Autodesk Fusion 360 part; units mm, degrees
sketch "Sketch1" plane through (0, 0, 0) normal (0, 0, 1) x (1, 0, 0)
  circle A0 centre (0, 0) radius 10
  dimension "d1" = 20
extrude "Extrude1" add sketch "Sketch1" along normal blind 3
sketch "Sketch2" plane through (0, 0, 3) normal (0, 0, 1) x (-1, 0, 0)
  circle A0 centre (0, 0) radius 10
  circle A1 centre (0, 0) radius 1.5
  dimension "d4" = 3
extrude "Extrude2" cut sketch "Sketch2" against normal blind 12 contours A1
sketch "Sketch3" plane through (0, 0, 3) normal (0, 0, 1) x (-1, 0, 0)
  circle A0 centre (0, 0) radius 1.5
  circle A1 centre (0, 0) radius 10
  circle A2 centre (-4.6093, 0.0139) radius 0.8
  dimension "d7" = 1.6
sketch "Sketch4" plane through (0, 0, 3) normal (0, 0, 1) x (-1, 0, 0)
  circle A0 centre (4.6091, 0) radius 0.8
  dimension "d8" = 1.6
extrude "Extrude3" cut sketch "Sketch3" sketch "Sketch4" against normal blind 3 contours A2 of sketch 2
CAD build for the part. Positions are in the model's coordinates, mm. Give positions to 0.01 mm unless a question says otherwise; leave off trailing zeros. Order: outer loops, then holes, each group sorted by start corner. A loop starts at its lowest first (then second) coordinate and runs counter-clockwise, first axis right, second up. Notation, with made-up numbers: (23.5, -11.75) - (46.5, -11.75) arc R18 cw to (46.5, -7.75) - close; hole circle Ø9 at (-17.75, -30). An arc over 180 degrees is marked (long way). Answer in a Markdown table with one row per item.
1. Flat gauge pin, fed straight in: pin 1 (1.3 mm diameter, centred on x = 4.61, y = -0.01, fed in from -Z). Where does the tip first touch, or does it go through?
Data:
| item | result |
|---|---|
| pin 1 | passes through |
2. Saw through at B-B, the plane y = 2.5. Give the cut face in (x, z), plus the area to 3 significant figures.
Data:
| item | result |
|---|---|
| outline | (-9.68, 0) - (9.68, 0) - (9.68, 3) - (-9.68, 3) - close |
| area | 58.1 mm² |
3. Probe probe 1 along Y at (x, z) = (0, 2.05); probe 2 along X at (y, z) = (-0.5, 1.8); probe 3 along Y at (x, z) = (1, 1.65). List the from-to ranges inside material, lowest first. Write a range as [from, to].
Data:
| item | result |
|---|---|
| probe 1 | y = [-10, -1.5], [1.5, 10] |
| probe 2 | x = [-9.99, -5.23], [-3.98, -1.41], [1.41, 3.97], [5.24, 9.99] |
| probe 3 | y = [-9.95, -1.12], [1.12, 9.95] |
4. Saw through at C-C, the plane z = 1.6. Give the cut face in (x, y), plus the area to 3 significant figures.
Data:
| item | result |
|---|---|
| outline | circle Ø20 at (0, 0); hole circle Ø1.6 at (-4.61, 0); hole circle Ø3 at (0, 0); hole circle Ø1.6 at (4.61, -0.01) |
| area | 303 mm² |
5. Saw through at D-D, the plane x = -6.25. Give the cut face in (y, z).
Data:
| item | result |
|---|---|
| outline | (-7.81, 0) - (7.81, 0) - (7.81, 3) - (-7.81, 3) - close |
6. Pull direction X, two halves, no side cores. Call faces 1 (the cylindrical face through (-2.17, 9.76, 1.48)), 2 (the cylindrical face through (1.5, -0.07, 1.52)), 3 (the flat face through (2, 0, 0)): pulls with the +X half, pulls with the -X half, needs draft (parallel to the pull), parting line crosses it, or undercut.
Data:
| item | result |
|---|---|
| face 1 | parting line crosses it |
| face 2 | undercut |
| face 3 | needs draft |
7. Saw through at A-A, the plane x = 0. Give the cut face in (y, z).
Data:
| item | result |
|---|---|
| outline | (-10, 0) - (-1.5, 0) - (-1.5, 3) - (-10, 3) - close; (1.5, 0) - (10, 0) - (10, 3) - (1.5, 3) - close |
